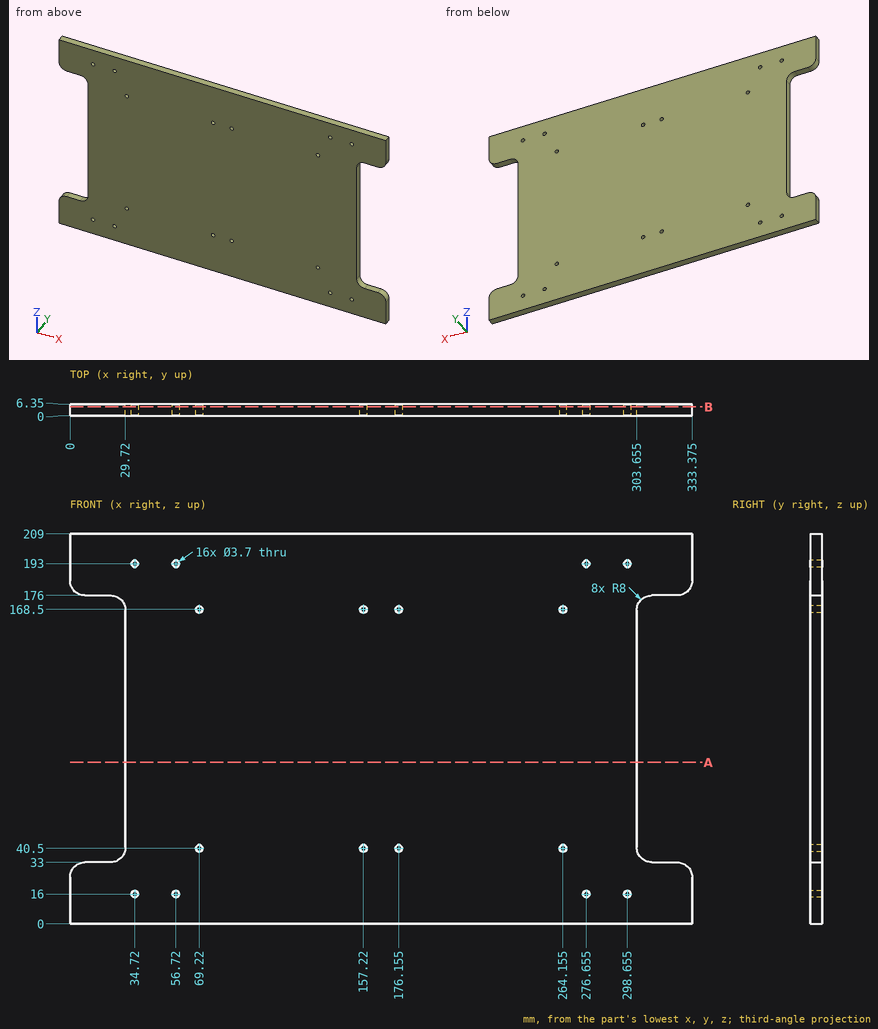
Could you check a few things on this drawing? It's one solid part, dimensions in mm from its lowest x, y, z. Round coordinates to 2 decimals unless told otherwise and drop trailing zeros. Write each loop counter-clockwise with the first axis right and the second up, starting at its lowest first coordinate (ties: lowest second). Pieces come first, ordered by that corner, then holes. Notation, with made-up numbers: (-10, 21) -> (21, 21) arc R17 ccw to (21, 44) -> close; hole circle Ø5 at (32.25, 6). An arc over 180 degrees is marked (long way). One line per question, with ' | ' between items. Start each with the question number.
1) I'm going to push flat-ended pins straight in: P1, Ø2, axis at x = 56.72, z = 193, coming from the -Y side; P2, Ø1.9, axis at y = 2, z = 123.5, coming from the -X side. Where does each tip first touch, or does it pass through?
2) Suppose I cut it at A-A on z = 86.5. Write out the boundary of the cut face in (x, y) (3 decimals), then the cut area to 3 significant figures.
3) Suppose I cut it at B-B on y = 4.75. Count the separate pieces of the cut face and the enclosed holes in it, then the cut area to 3 significant figures.
4) I need wall thicknesses on line 1 (X direction, y = 3, z = 40.5) (3 decimals); line 2 (X direction, y = 4, z = 16) (3 decimals); line 3 (Z direction, x = 298.5, y = 0.5). Which ranges of each line are inside material? Lowest first, please. Write a range as [from, to].
Return value:
1) P1: passes through | P2: stops at x = 29.72
2) outline: (29.72, 0) -> (303.655, 0) -> (303.655, 6.35) -> (29.72, 6.35) -> close | area: 1,740 mm2
3) separate pieces: 1 | enclosed holes: 16 | area: 61,000 mm2
4) line 1: x = [29.704, 67.37], [71.07, 155.37], [159.07, 174.305], [178.005, 262.305], [266.005, 303.671] | line 2: x = [0, 32.87], [36.57, 54.87], [58.57, 274.805], [278.505, 296.805], [300.505, 333.375] | line 3: z = [0, 14.16], [17.84, 191.16], [194.84, 209]
